Verification items for the finished model (mm, model axes). Face numbers are marked on the shaded views. A direction names the side the tool comes from. Give positions to 0.01 mm unless a question says otherwise; leave off trailing zeros. Loops run counter-clockwise (first coordinate to the right, second up) from the corner with the lowest first, then second, coordinate; pieces in that order, holes last. Notation, with made-up numbers: (18.5, -19) - (71.5, -19) arc R23 ccw to (71.5, -11) - close; hole circle Ø6 at (46.5, -16.75). An arc over 180 degrees is marked (long way). Use one line per item in the form item = value.
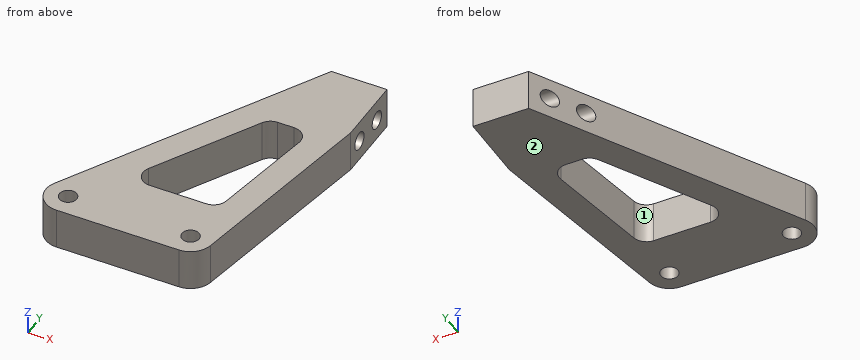
```python
from build123d import *

# Parameters (mm, degrees)
BOSS_EXTRUDE1_DEPTH = 7.5
SKETCH2_R           = 1.55
CUT_EXTRUDE1_DEPTH  = 18.24093965
BOSS_EXTRUDE6_START = -7.5
BOSS_EXTRUDE6_DEPTH = 7.5
CUT_EXTRUDE2_REACH  = 62.49
SKETCH13_R          = 1.6
CUT_EXTRUDE8_DEPTH  = 53.848740761
FILLET1_R           = 2.5


with BuildPart() as part:
    # Sketch1 → Boss-Extrude1 (new body)
    with BuildSketch(Plane.XY):
        with BuildLine():
            Line((-11, 4), (11, 4))
            ThreePointArc((11, 4), (15, 0), (11, -4))
            Line((11, -4), (-11, -4))
            ThreePointArc((-11, -4), (-15, 0), (-11, 4))
        make_face()
    extrude(amount=BOSS_EXTRUDE1_DEPTH)

    # Sketch2 → Cut-Extrude1 (cut, through all)
    with BuildSketch(Plane.XY.offset(7.5)):
        with Locations((-11, 0)):
            Circle(SKETCH2_R)
    cut_extrude1 = extrude(amount=-CUT_EXTRUDE1_DEPTH, mode=Mode.SUBTRACT)

    # Mirror1: Cut-Extrude1 across plane
    add(cut_extrude1.mirror(Plane(origin=(0, 0, 0), x_dir=(0, 0, 1), z_dir=(1, 0, 0))), mode=Mode.SUBTRACT)

    # Sketch12 → Boss-Extrude6 (add)
    with BuildSketch(Plane.XY.offset(7.5).offset(BOSS_EXTRUDE6_START)):
        with BuildLine():
            Line((21.37, 35.25), (21.37, 47.75))
            Line((21.37, 47.75), (11.37, 47.75))
            Line((11.37, 47.75), (-14.48304631, 1.966821905))
            ThreePointArc((-14.48304631, 1.966821905), (-13.016520813, 3.454510647), (-11, 4))
            Line((-11, 4), (11, 4))
            ThreePointArc((11, 4), (14.067391334, 2.567315797), (14.937481114, -0.704444799))
            Line((14.937481114, -0.704444799), (21.37, 35.25))
        make_face()
    extrude(amount=BOSS_EXTRUDE6_DEPTH)

    # Cut-Extrude2: up to this plane
    cut_extrude2_end = Plane(origin=(-11.823529281, 6.676562501, -60.276646808), z_dir=(-0.870761577419204, 0.49170547616476634, 0))
    # Sketch13 → Cut-Extrude2 (cut, up to the surface)
    with BuildSketch(Plane(origin=(21.37, 0, 0), x_dir=(0, 0, -1), z_dir=(1, 0, 0)), mode=Mode.PRIVATE) as cut_extrude2_sk1:
        with Locations((-3.75, 38.25)):
            Circle(SKETCH13_R)
    cut_extrude2_tool1 = split(extrude(cut_extrude2_sk1.sketch, amount=-CUT_EXTRUDE2_REACH, mode=Mode.PRIVATE), bisect_by=cut_extrude2_end, keep=Keep.BOTH, mode=Mode.PRIVATE)
    add(cut_extrude2_tool1.solids().sort_by_distance((21.37, 38.25, 3.75))[0], mode=Mode.SUBTRACT)
    # Sketch13 → Cut-Extrude2 (cut, up to the surface)
    with BuildSketch(Plane(origin=(21.37, 0, 0), x_dir=(0, 0, -1), z_dir=(1, 0, 0)), mode=Mode.PRIVATE) as cut_extrude2_sk2:
        with Locations((-3.75, 44.25)):
            Circle(SKETCH13_R)
    cut_extrude2_tool2 = split(extrude(cut_extrude2_sk2.sketch, amount=-CUT_EXTRUDE2_REACH, mode=Mode.PRIVATE), bisect_by=cut_extrude2_end, keep=Keep.BOTH, mode=Mode.PRIVATE)
    add(cut_extrude2_tool2.solids().sort_by_distance((21.37, 44.25, 3.75))[0], mode=Mode.SUBTRACT)

    # Sketch15 → Cut-Extrude8 (cut, through all)
    with BuildSketch(Plane.XY.offset(7.5)):
        Polygon((15.753888137, 32.25), (8.359491787, 32.25), (-5.051762639, 8.5), (11.504835638, 8.5), align=None)
    extrude(amount=-CUT_EXTRUDE8_DEPTH, mode=Mode.SUBTRACT)

    # Fillet1
    fillet1_edges = [part.edges().sort_by_distance(p)[0] for p in [
        (8.359491787, 32.25, 3.75),
        (15.753888137, 32.25, 3.75),
        (11.504835638, 8.5, 3.75),
        (-5.051762639, 8.5, 3.75),
    ]]
    fillet(fillet1_edges, radius=FILLET1_R)


solid = part.part
```
1. Section check D-D, the plane y = 0. Record the cut outline in (x, z), then the cut area to 3 significant figures.
Result set:
outline = (-15, 0) - (-12.55, 0) - (-12.55, 7.5) - (-15, 7.5) - close; (-9.45, 0) - (9.45, 0) - (9.45, 7.5) - (-9.45, 7.5) - close; (12.55, 0) - (15.06, 0) - (15.06, 7.5) - (12.55, 7.5) - close
area = 179 mm²
2. Depth check by flat-ended pin: pin 1 Ø3 at (x, y) = (11, 0) entering from -Z; pin 2 Ø3 at (y, z) = (5, 6.5) entering from -X; pin 3 Ø2 at (x, z) = (2, 3.5) entering from +Y. Enter the tip coordinate at first touch or a pass-through.
Result set:
pin_1 = through
pin_2 = -13.62
pin_3 = 32.93
3. Section check B-B, the plane y = 20.5. Record the cut outline in (x, z).
Result set:
outline = (-4.02, 0) - (1.72, 0) - (1.72, 7.5) - (-4.02, 7.5) - close; (13.65, 0) - (18.73, 0) - (18.73, 7.5) - (13.65, 7.5) - close
4. Tool access check on the marked faces 1 and 2. Record the directions out of +Z, -Z, +X, -X, +Y, -Y that give a thin tool (end or side, any length) a straight path to the whole face; none if there is none.
Result set:
face_1 = +Z, -Z
face_2 = -Z, +X, -X, +Y, -Y
5. Scan lines: probe 1 along Y at (x, z) = (11, 3); probe 2 along Y at (x, z) = (10, 1); probe 3 along Z at (x, y) = (11, 38.25). Record each from-to range of solid material in increasing order.
Result set:
probe_1 = -4 to -1.55, 1.55 to 9.07, 32.25 to 36.84, 39.66 to 42.84, 45.66 to 47.09
probe_2 = -4 to -1.18, 1.18 to 8.57, 32.25 to 45.32
probe_3 = 0 to 2.15, 5.35 to 7.5
6. Section check A-A, the plane z = 6.5. Record the cut outline in (x, y), then the cut area to 3 significant figures.
Result set:
outline = (-14.48, 1.97) arc R4 ccw to (-11, -4) - (11, -4) arc R4 ccw to (14.94, -0.7) - (21.37, 35.25) - (21.37, 47.75) - (11.37, 47.75) - close; hole circle Ø3.1 at (-11, 0); hole (-2.95, 12.23) arc R2.5 ccw to (-0.77, 8.5) - (9.41, 8.5) arc R2.5 ccw to (11.87, 10.56) - (15.23, 29.31) arc R2.5 ccw to (12.77, 32.25) - (9.82, 32.25) arc R2.5 ccw to (7.64, 30.98) - close; hole circle Ø3.1 at (11, 0)
area = 831 mm²
7. Section check C-C, the plane z = 4. Record the cut outline in (x, y), then the cut area to 3 significant figures.
Result set:
outline = (-14.48, 1.97) arc R4 ccw to (-11, -4) - (11, -4) arc R4 ccw to (14.94, -0.7) - (21.37, 35.25) - (21.37, 36.67) - (5.11, 36.67) - close; (6.9, 39.83) - (21.37, 39.83) - (21.37, 42.67) - (8.5, 42.67) - close; (10.29, 45.83) - (21.37, 45.83) - (21.37, 47.75) - (11.37, 47.75) - close; hole circle Ø3.1 at (-11, 0); hole (-2.95, 12.23) arc R2.5 ccw to (-0.77, 8.5) - (9.41, 8.5) arc R2.5 ccw to (11.87, 10.56) - (15.23, 29.31) arc R2.5 ccw to (12.77, 32.25) - (9.82, 32.25) arc R2.5 ccw to (7.64, 30.98) - close; hole circle Ø3.1 at (11, 0)
area = 744 mm²
